```python
from build123d import *

# Parameters (mm, degrees)
SKETCH1_W            = 66
SKETCH1_H            = 30
BOSS_EXTRUDE1_DEPTH  = 56
CHAMFER1_SIZE        = 1
SKETCH3_W            = 8.5
SKETCH3_H            = 30
BOSS_EXTRUDE2_DEPTH  = 4
CUT_EXTRUDE1_REACH   = 87.86
BOSS_EXTRUDE3_DEPTH  = 1.5
FILLET2_R            = 1.5
FILLET2_OF_MIRROR1_R = 1.5
CUT_EXTRUDE2_DEPTH   = 5.5
FILLET3_R            = 1.5
BOSS_EXTRUDE4_DEPTH  = 2
FILLET4_R            = 1
SKETCH8_R            = 9
BOSS_EXTRUDE5_DEPTH  = 3.2
SKETCH9_R            = 7
BOSS_EXTRUDE6_DEPTH  = 0.5
BOSS_EXTRUDE8_DEPTH  = 5.5
CIRPATTERN1_COUNT    = 15


with BuildPart() as part:
    # Sketch1 → Boss-Extrude1 (new body)
    with BuildSketch(Plane(origin=(0, 0, 0), x_dir=(1, 0, 0), z_dir=(0, 1, 0))):
        with Locations((33, 15)):
            Rectangle(SKETCH1_W, SKETCH1_H)
    extrude(amount=BOSS_EXTRUDE1_DEPTH)

    # Chamfer1
    chamfer1_edges = [part.edges().sort_by_distance(p)[0] for p in [
        (33, 0, -30),
        (66, 0, -15),
        (33, 0, 0),
        (0, 0, -15),
    ]]
    chamfer(chamfer1_edges, length=CHAMFER1_SIZE)

    # Sketch3 → Boss-Extrude2 (add)
    with BuildSketch(Plane(origin=(0, 42, 0), x_dir=(1, 0, 0), z_dir=(0, 1, 0))):
        with Locations((-4.25, 15)):
            Rectangle(SKETCH3_W, SKETCH3_H)
    boss_extrude2 = extrude(amount=BOSS_EXTRUDE2_DEPTH)

    # Sketch4 → Cut-Extrude1 (cut, up to next)
    with BuildSketch(Plane(origin=(0, 46, 0), x_dir=(1, 0, 0), z_dir=(0, 1, 0)), mode=Mode.PRIVATE) as cut_extrude1_sk1:
        with BuildLine():
            Line((-8.5, 8), (-6.621320344, 8))
            ThreePointArc((-6.621320344, 8), (-1.75, 6.25), (-6.621320344, 4.5))
            Line((-6.621320344, 4.5), (-8.5, 4.5))
            Line((-8.5, 4.5), (-8.5, 8))
        make_face()
    cut_extrude1_tool1 = extrude(cut_extrude1_sk1.sketch, amount=-CUT_EXTRUDE1_REACH, mode=Mode.PRIVATE) & part.part
    # Sketch4 → Cut-Extrude1 (cut, up to next)
    with BuildSketch(Plane(origin=(0, 46, 0), x_dir=(1, 0, 0), z_dir=(0, 1, 0)), mode=Mode.PRIVATE) as cut_extrude1_sk2:
        with BuildLine():
            Line((-8.5, 25.5), (-6.621320344, 25.5))
            ThreePointArc((-6.621320344, 25.5), (-1.75, 23.75), (-6.621320344, 22))
            Line((-6.621320344, 22), (-8.5, 22))
            Line((-8.5, 22), (-8.5, 25.5))
        make_face()
    cut_extrude1_tool2 = extrude(cut_extrude1_sk2.sketch, amount=-CUT_EXTRUDE1_REACH, mode=Mode.PRIVATE) & part.part
    cut_extrude1_1 = cut_extrude1_tool1.solids().sort_by_distance((-5.074136, 46, -6.25))[0]
    add(cut_extrude1_1, mode=Mode.SUBTRACT)
    cut_extrude1_2 = cut_extrude1_tool2.solids().sort_by_distance((-5.074136, 46, -23.75))[0]
    add(cut_extrude1_2, mode=Mode.SUBTRACT)
    cut_extrude1 = cut_extrude1_1 + cut_extrude1_2  # Cut-Extrude1 as one shape, for the pattern or mirror that repeats it

    # Sketch5 → Boss-Extrude3 (add, symmetric)
    with BuildSketch(Plane.XY.offset(-15)):
        Polygon((-8.5, 46), (0, 46), (0, 48), (-5.5, 48), align=None)
    boss_extrude3 = extrude(amount=BOSS_EXTRUDE3_DEPTH, both=True)

    # Fillet2
    fillet2_edges = [part.edges().sort_by_distance(p)[0] for p in [
        (-8.5, 44, -30),
        (-8.5, 44, 0),
    ]]
    fillet(fillet2_edges, radius=FILLET2_R)

    # Mirror1: Boss-Extrude2, Cut-Extrude1, Boss-Extrude3 across plane
    add(boss_extrude2.mirror(Plane.ZY.offset(-33)))
    add(cut_extrude1.mirror(Plane.ZY.offset(-33)), mode=Mode.SUBTRACT)
    add(boss_extrude3.mirror(Plane.ZY.offset(-33)))

    # Fillet2 of Mirror1
    fillet2_of_mirror1_edges = [part.edges().sort_by_distance(p)[0] for p in [
        (74.5, 44, -30),
        (74.5, 44, 0),
    ]]
    fillet(fillet2_of_mirror1_edges, radius=FILLET2_OF_MIRROR1_R)

    # Sketch6 → Cut-Extrude2 (cut)
    with BuildSketch(Plane(origin=(0, 56, 0), x_dir=(1, 0, 0), z_dir=(0, 1, 0))):
        with BuildLine():
            Line((13.5, 0), (13.5, 8))
            ThreePointArc((13.5, 8), (6.738519216, 13.188266684), (10, 21.062177826))
            Line((10, 21.062177826), (10, 30))
            Line((10, 30), (0, 30))
            Line((0, 30), (0, 0))
            Line((0, 0), (13.5, 0))
        make_face()
    extrude(amount=-CUT_EXTRUDE2_DEPTH, mode=Mode.SUBTRACT)

    # Fillet3
    fillet3_edges = [part.edges().sort_by_distance(p)[0] for p in [
        (66, 21.5, 0),
        (66, 21.5, -30),
        (0, 48.25, -30),
        (0, 48.25, 0),
        (10, 53.25, -30),
        (13.5, 53.25, 0),
        (0, 21.5, -30),
        (0, 21.5, 0),
        (66, 51, -30),
        (66, 51, 0),
    ]]
    fillet(fillet3_edges, radius=FILLET3_R)

    # Sketch7 → Boss-Extrude4 (add)
    with BuildSketch(Plane(origin=(0, 56, 0), x_dir=(1, 0, 0), z_dir=(0, 1, 0))):
        with BuildLine():
            Line((13.5, 9), (37, 9))
            Line((37, 9), (37, 29))
            Line((37, 29), (11, 29))
            Line((11, 29), (11, 20.454356057))
            ThreePointArc((11, 20.454356057), (7.637997938, 13.720573633), (13.5, 9))
        make_face()
    extrude(amount=BOSS_EXTRUDE4_DEPTH)

    # Fillet4
    fillet4_edges = [part.edges().sort_by_distance(p)[0] for p in [
        (37, 57, -9),
        (37, 57, -29),
        (11, 57, -29),
    ]]
    fillet(fillet4_edges, radius=FILLET4_R)

    # Sketch8 → Boss-Extrude5 (add)
    with BuildSketch(Plane(origin=(0, 56, 0), x_dir=(1, 0, 0), z_dir=(0, 1, 0))):
        with Locations(Location((51, 15, 0), (0, 0, 90))):
            Circle(SKETCH8_R)
    extrude(amount=BOSS_EXTRUDE5_DEPTH)

    # Sketch9 → Boss-Extrude6 (add)
    with BuildSketch(Plane(origin=(0, 59.2, 0), x_dir=(1, 0, 0), z_dir=(0, 1, 0))):
        with Locations(Location((51, 15, 0), (0, 0, 270))):
            Circle(SKETCH9_R)
    extrude(amount=BOSS_EXTRUDE6_DEPTH)

    # Sketch10 → Boss-Extrude8 (add)
    with BuildSketch(Plane(origin=(0, 59.7, 0), x_dir=(1, 0, 0), z_dir=(0, 1, 0))):
        Polygon((50.25, 17.928888995), (51, 19), (51.75, 17.928888995), (51.75, 15), (50.25, 15), align=None)
    boss_extrude8 = extrude(amount=BOSS_EXTRUDE8_DEPTH)

    # CirPattern1: Boss-Extrude8 ×15 about axis
    cirpattern1_axis = Axis((51, 0, -15), (0, 1, 0))
    for i in range(1, CIRPATTERN1_COUNT):
        add(boss_extrude8.rotate(cirpattern1_axis, i * 360 / CIRPATTERN1_COUNT))

    # Sketch13 → Cut-Revolve1 (revolve, cut)
    with BuildSketch(Plane(origin=(51, 0, 0), x_dir=(0, -1, 0), z_dir=(-1, 0, 0))):
        Polygon((-65.2, -18.2), (-65.2, -19), (-64.4, -19), align=None)
    revolve(axis=Axis((51, 66.624672481, -15), (0, -1, 0)), mode=Mode.SUBTRACT)


solid = part.part
```
Design review of the part built by this model. Coordinates are the model's own, in mm. A direction names the side the tool comes from. Coordinates: 2 decimals unless noted, no trailing zeros. Order: outer loops, then holes, each group sorted by start corner. A loop starts at its lowest first (then second) coordinate and runs counter-clockwise, first axis right, second up. Notation, with made-up numbers: (1.5, -31) - (24.5, -31) arc R16 cw to (24.5, -20) - close; hole circle Ø4 at (69, 73.5). An arc over 180 degrees is marked (long way). One line per question, with ' | ' between items.
Q1. The part is to be moulded in two halves that separate along Z. For faces 1 (the flat face through (-3, 47, -13.5)), 2 (the flat face through (-8, 44, -22)), 3 (the flat face through (69, 47, -16.5)), 4 (the flat face through (10, 53, -25)), say which applies: +Z half, -Z half, draft (parallel to the pull), parting line (faces both ways), or undercut.
Answer key:
face 1: +Z half | face 2: undercut | face 3: -Z half | face 4: draft
Q2. Consider section D-D, the plane x = 9. Give the boundary of the cut face in (y, z), then the cut area to 3 significant figures.
Answer key:
outline: (0, -29) - (1, -30) - (50.5, -30) - (50.5, -20.36) - (56, -20.36) - (56, -18.97) - (58, -18.97) - (58, -11.03) - (56, -11.03) - (56, -9.64) - (50.5, -9.64) - (50.5, 0) - (1, 0) - (0, -1) - close | area: 1,590 mm2
Q3. Consider section A-A, the plane x = 70.5. Give the boundary of the cut face in (y, z), then the cut area to 3 significant figures.
Answer key:
outline: (42, -30) - (46, -30) - (46, -26.5) - (42, -26.5) - close; (42, -21) - (46, -21) - (46, -16.5) - (48, -16.5) - (48, -13.5) - (46, -13.5) - (46, -9) - (42, -9) - close; (42, -3.5) - (46, -3.5) - (46, 0) - (42, 0) - close | area: 82.0 mm2
Q4. Clearance check with flat-ended pins moving along their axes: pin 1 Ø1 at (x, z) = (16, -7) entering from +Y; pin 2 Ø6 at (y, z) = (53, -24) entering from -X; pin 3 Ø13.5 at (y, z) = (15.5, -14) entering from +X; pin 4 Ø4.5 at (x, z) = (-4.5, -23.75) entering from -Y. State where each tip first meets the part, or that it passes through.
Answer key:
pin 1: stops at y = 56 | pin 2: stops at x = 0 | pin 3: stops at x = 66 | pin 4: passes through
Q5. Consider section B-B, the plane y = 40.5. Give the boundary of the cut face in (x, z), then the cut area to 3 significant figures.
Answer key:
outline: (0, -28.5) arc R1.5 ccw to (1.5, -30) - (64.5, -30) arc R1.5 ccw to (66, -28.5) - (66, -1.5) arc R1.5 ccw to (64.5, 0) - (1.5, 0) arc R1.5 ccw to (0, -1.5) - close | area: 1,980 mm2
Q6. For faces 5 (the flat face through (-3, 48, -15)), 6 (the flat face through (69, 48, -15)), 7 (the cylindrical face through (6.773, 53.288, -13.065)), 8 (the flat face through (13.5, 53, -5)), 9 (the flat face through (66, 21, -15)), list the 3-axis set-ups (+Z, -Z, +X, -X, +Y, -Y) from which the entire face can be reached by the end or side of a thin tool; tool diameter is ignored.
Answer key:
face 5: +Z, -Z, -X, +Y | face 6: +Z, -Z, +X, +Y | face 7: -X, +Y | face 8: +Z, -X, +Y | face 9: +Z, -Z, +X, -Y
Q7. To check wall thickness, follow line 1 along Z through (x, y) = (-4.5, 45.05); line 2 along X through (y, z) = (44.5, -4.25); line 3 along X through (y, z) = (43.9, -23.75). State the ranges of each line that lie inside material, in increasing order.
Answer key:
line 1: z = -30 to -26.5, -21 to -9, -3.5 to 0 | line 2: x = -8.5 to -6.39, -2.61 to 68.61, 72.39 to 74.5 | line 3: x = -1.75 to 67.75
Q8. Consider section C-C, the plane z = -7. Give the boundary of the cut face in (x, y).
Answer key:
outline: (-1.85, 42) - (0, 42) - (0, 1) - (1, 0) - (65, 0) - (66, 1) - (66, 42) - (67.85, 42) - (67.85, 46) - (66, 46) - (66, 56) - (55.12, 56) - (55.12, 59.2) - (46.88, 59.2) - (46.88, 56) - (13.5, 56) - (13.5, 50.5) - (0, 50.5) - (0, 46) - (-1.85, 46) - close
